Check sheet for the modelled part. Datum: model origin and axes. Units: mm. Give positions to 0.01 mm unless a question says otherwise; leave off trailing zeros. Write each loop counter-clockwise with the first axis right and the second up, starting at its lowest first coordinate (ties: lowest second). Pieces come first, ordered by that corner, then holes. Notation, with made-up numbers: (-6, 4.25) -> (40, 4.25) arc R31 ccw to (40, 30.25) -> close; hole circle Ø11 at (16, 50). An arc over 180 degrees is marked (long way). Use a Markdown table: item, result. Add a question column.
1. Gauge pin test, flat end, axial feed: P1, Ø1, axis at x = -1, z = 0.5, coming from the +Y side. Record the tip position at first contact, or that the pin passes through.
2. Scan lines: probe 1 along Y at (x, z) = (0, 0.6); probe 2 along X at (y, z) = (-1, 0.6); probe 3 along Y at (x, z) = (1, 2.95). Record each from-to range of solid material in increasing order. Write a range as [from, to].
3. Cross-section at C-C (z = 0.7). Enter the section's corners in (x, y).
4. Release check for a two-part mould opening along X. For faces 1 (the cylindrical face through (2, 0, 1)), 2 (the flat face through (-2, -3, 3)), 3 (the cylindrical face through (-0.867, 3.905, 1.479)) record: released by +X, released by -X, zero draft, split by the parting line, or undercut.
5. Cross-section at A-A (x = 0). Enter the section's corners in (y, z) (3 decimals), then the cut area to 3 significant figures.
Autodesk Fusion 360 part; units mm, degrees
sketch "Sketch1" plane through (0, 0, 0) normal (0, 0, 1) x (1, 0, 0)
  circle A0 centre (0, 0) radius 3.5
  circle A1 centre (0, 0) radius 1.6
  dimension "d1" = 7
  dimension "d2" = 3.2
extrude "Extrude1" add sketch "Sketch1" along normal blind 0.5

Autodesk Fusion 360 part; units mm, degrees
sketch "Sketch1" plane through (0, 0, 0) normal (0, 0, 1) x (1, 0, 0)
  circle A0 centre (0, 0) radius 4
  dimension "d1" = 8
extrude "Extrude1" add sketch "Sketch1" along normal blind 3
hole "Hole1" at (0, 0, 3) direction (0, 0, -1) diameter 4 end through all countersink diameter 6.75 countersink angle 90
Worked answers:
| question | item | result |
|---|---|---|
| 1 | P1 | stops at y = 3.97 |
| 2 | probe 1 | y = [-4, -2], [2, 4] |
| 2 | probe 2 | x = [-3.87, -1.73], [1.73, 3.87] |
| 2 | probe 3 | y = [-3.87, -3.17], [3.17, 3.87] |
| 3 | outline | circle Ø8 at (0, 0); hole circle Ø4 at (0, 0) |
| 4 | face 1 | undercut |
| 4 | face 2 | zero draft |
| 4 | face 3 | split by the parting line |
| 5 | outline | (-4, 0) -> (-2, 0) -> (-2, 1.625) -> (-3.375, 3) -> (-4, 3) -> close; (2, 0) -> (4, 0) -> (4, 3) -> (3.375, 3) -> (2, 1.625) -> close |
| 5 | area | 10.1 mm² |
